```python
from build123d import *

# Parameters (mm, degrees)
BOSS_EXTRUDE1_DEPTH        = 55
BOSS_EXTRUDE1_DEPTH_BACK   = 5
SKETCH1_R                  = 40
SKETCH1_R_2                = 30
SKETCH2_R                  = 10
SKETCH2_R_2                = 30
BOSS_EXTRUDE2_DEPTH        = 30
FILLET1_R                  = 20
SKETCH3_W                  = 60
SKETCH3_H                  = 20
CUT_EXTRUDE1_DEPTH         = 25
M10X1_0_TAPPED_HOLE1_D     = 9
M10X1_0_TAPPED_HOLE1_DEPTH = 43
M10X1_0_TAPPED_HOLE1_TIP   = 2.703872786


with BuildPart() as part:
    # Sketch1 → Boss-Extrude1 (new, two sides: drawn at the far end of the back side and taken through both)
    with BuildSketch(Plane(origin=(0, 0, 0), x_dir=(1, 0, 0), z_dir=(0, 1, 0)).offset(-BOSS_EXTRUDE1_DEPTH_BACK)):
        with Locations(Location((0, 0, 0), (0, 0, 270))):
            Circle(SKETCH1_R)
        with Locations(Location((0, 0, 0), (0, 0, 270))):
            Circle(SKETCH1_R_2, mode=Mode.SUBTRACT)
    extrude(amount=BOSS_EXTRUDE1_DEPTH + BOSS_EXTRUDE1_DEPTH_BACK)

    # Sketch2 → Boss-Extrude2 (add)
    with BuildSketch(Plane(origin=(0, 0, 0), x_dir=(1, 0, 0), z_dir=(0, 1, 0))):
        with BuildLine():
            Line((39.875, -37.881187613), (71.35896205, -19.999349518))
            ThreePointArc((71.35896205, -19.999349518), (83, 0), (71.35896205, 19.999349518))
            Line((71.35896205, 19.999349518), (39.875, 37.881187613))
            Line((39.875, 37.881187613), (35, 40.650024667))
            Line((35, 40.650024667), (35, 72.426406871))
            Line((35, 72.426406871), (-35, 72.426406871))
            Line((-35, 72.426406871), (-35, 40.650024667))
            Line((-35, 40.650024667), (-39.875, 37.881187613))
            Line((-39.875, 37.881187613), (-71.35896205, 19.999349518))
            ThreePointArc((-71.35896205, 19.999349518), (-83, 0), (-71.35896205, -19.999349518))
            Line((-71.35896205, -19.999349518), (-39.875, -37.881187613))
            ThreePointArc((-39.875, -37.881187613), (0, -55), (39.875, -37.881187613))
        make_face()
        with Locations(Location((-60, 0, 0), (0, 0, 270))):
            Circle(SKETCH2_R, mode=Mode.SUBTRACT)
        with Locations(Location((0, 0, 0), (0, 0, 270))):
            Circle(SKETCH2_R_2, mode=Mode.SUBTRACT)
        with Locations(Location((60, 0, 0), (0, 0, 270))):
            Circle(SKETCH2_R, mode=Mode.SUBTRACT)
    extrude(amount=BOSS_EXTRUDE2_DEPTH)

    # Fillet1
    fillet1_edges = [part.edges().sort_by_distance(p)[0] for p in [
        (35, 15, -40.650024667),
        (-35, 15, -40.650024667),
    ]]
    fillet(fillet1_edges, radius=FILLET1_R)

    # Sketch3 → Cut-Extrude1 (cut)
    with BuildSketch(Plane(origin=(0, 0, -72.426406871), x_dir=(-1, 0, 0), z_dir=(0, 0, -1))):
        with Locations((0, 15)):
            Rectangle(SKETCH3_W, SKETCH3_H)
    extrude(amount=-CUT_EXTRUDE1_DEPTH, mode=Mode.SUBTRACT)

    # M10x1.0 Tapped Hole1
    with Locations(Plane(origin=(0, 15, -47.426406871), x_dir=(-1, 0, 0), z_dir=(0, 0, -1))):
        with Locations((0, 0)):
            Hole(M10X1_0_TAPPED_HOLE1_D / 2, depth=M10X1_0_TAPPED_HOLE1_DEPTH)
            with Locations((0, 0, -(M10X1_0_TAPPED_HOLE1_DEPTH + M10X1_0_TAPPED_HOLE1_TIP / 2))):  # 118° drill point
                Cone(0, M10X1_0_TAPPED_HOLE1_D / 2, M10X1_0_TAPPED_HOLE1_TIP, mode=Mode.SUBTRACT)


solid = part.part
```
Geometry: final body of the model. Coordinates: model frame, mm. A direction names the side the tool comes from. Round coordinates to 2 decimals unless told otherwise and drop trailing zeros. Order: outer loops, then holes, each group sorted by start corner. A loop starts at its lowest first (then second) coordinate and runs counter-clockwise, first axis right, second up. Notation, with made-up numbers: (74.25, 65) -> (93.25, 65) arc R11 cw to (93.25, 85) -> close; hole circle Ø10 at (58.5, 30). An arc over 180 degrees is marked (long way). Write each question's results on one line, items separated by ' | '.
Q1. Pull-direction query (X, two-part tool) for faces 1 (the face through (-58.057, 14.79, -27.554)), 2 (the face through (0.5, 4.8, -72.426)), 3 (the face through (2.419, 18.794, -38.419)); classes: released by +X, released by -X, zero draft, split by the parting line, or undercut.
Response values:
face 1: released by -X | face 2: zero draft | face 3: undercut
Q2. Section query B-B (x = 0). Output: boundary loops of the cut face in (y, z), and give its area (3 significant figures).
Response values:
outline: (-5, -40) -> (0, -40) -> (0, -72.43) -> (5, -72.43) -> (5, -47.43) -> (10.5, -47.43) -> (10.5, -30) -> (-5, -30) -> close; (-5, 30) -> (55, 30) -> (55, 40) -> (30, 40) -> (30, 55) -> (0, 55) -> (0, 40) -> (-5, 40) -> close; (19.5, -47.43) -> (25, -47.43) -> (25, -72.43) -> (30, -72.43) -> (30, -40) -> (55, -40) -> (55, -30) -> (19.5, -30) -> close | area: 1,970 mm²
Q3. Ray query, line 1 along X through (y, z) = (22.25, 0); line 2 along X through (y, z) = (19, -65.5); line 3 along X through (y, z) = (29.5, -5). Return the intervals inside material, ascending.
Response values:
line 1: -83 to -70, -50 to -30, 30 to 50, 70 to 83 | line 2: -35 to -30, 30 to 35 | line 3: -82.45 to -68.66, -51.34 to -29.58, 29.58 to 51.34, 68.66 to 82.45
Q4. Section query D-D (x = 17). Output: boundary loops of the cut face in (y, z), and give its area (3 significant figures).
Response values:
outline: (-5, -36.21) -> (0, -36.21) -> (0, -72.43) -> (5, -72.43) -> (5, -47.43) -> (25, -47.43) -> (25, -72.43) -> (30, -72.43) -> (30, -36.21) -> (55, -36.21) -> (55, -24.72) -> (-5, -24.72) -> close; (-5, 24.72) -> (55, 24.72) -> (55, 36.21) -> (30, 36.21) -> (30, 52.31) -> (0, 52.31) -> (0, 36.21) -> (-5, 36.21) -> close | area: 2,450 mm²
Q5. Access query for faces 4 (the face through (-35, 15, -62)), 5 (the face through (30, 15, -60)), 6 (the face through (17, 30, -38)), 7 (the face through (17, 0, -38)). Directions: +Z, -Z, +X, -X, +Y, -Y. A direction counts if a zero-diameter tool reaches every point of the face in a straight line with its end or side. Return the directions, or none.
Response values:
face 4: -Z, -X, +Y, -Y | face 5: -Z | face 6: +Y | face 7: -Y
Q6. Section query C-C (z = -60). Output: boundary loops of the cut face in (x, y), and give its area (3 significant figures).
Response values:
outline: (-35, 0) -> (35, 0) -> (35, 30) -> (-35, 30) -> close; hole (-30, 5) -> (30, 5) -> (30, 25) -> (-30, 25) -> close | area: 900 mm²
Q7. Pin query (flat end, axial travel): pin 1 Ø18 at (x, z) = (-60, 0) entering from +Y (3 decimals); pin 2 Ø16 at (x, y) = (5, 11.5) entering from -Z; pin 3 Ø6 at (y, z) = (21, -59.5) entering from +X; pin 4 Ø4 at (y, z) = (1.5, -34.5) entering from +X. Return the tip coordinate at first contact, or that it passes through.
Response values:
pin 1: through | pin 2: z = -72.43 | pin 3: x = 35 | pin 4: x = 49.35
Q8. Section query A-A (z = 0). Output: boundary loops of the cut face in (x, y), and give its area (3 significant figures).
Response values:
outline: (-83, 0) -> (-70, 0) -> (-70, 30) -> (-83, 30) -> close; (-50, 0) -> (-40, 0) -> (-40, -5) -> (-30, -5) -> (-30, 55) -> (-40, 55) -> (-40, 30) -> (-50, 30) -> close; (30, -5) -> (40, -5) -> (40, 0) -> (50, 0) -> (50, 30) -> (40, 30) -> (40, 55) -> (30, 55) -> close; (70, 0) -> (83, 0) -> (83, 30) -> (70, 30) -> close | area: 2,580 mm²
